```python
from build123d import *

# Parameters (mm, degrees)
BOSS_EXTRUDE1_DEPTH = 5
SKETCH2_R           = 11.25
CUT_EXTRUDE1_DEPTH  = 2.5
SKETCH3_R           = 1.5
SKETCH3_R_2         = 1
CUT_EXTRUDE3_DEPTH  = 12.5
CHAMFER1_SIZE       = 2.5
SKETCH5_R           = 5
CUT_EXTRUDE4_DEPTH  = 12.5


with BuildPart() as part:
    # Sketch1 → Boss-Extrude1 (new body)
    with BuildSketch(Plane(origin=(0, 0, 0), x_dir=(1, 0, 0), z_dir=(0, 1, 0))):
        Polygon((-65, 2.5), (-65, -17.5), (65, -17.5), (65, 2.5), (50, 17.5), (-50, 17.5), align=None)
    extrude(amount=BOSS_EXTRUDE1_DEPTH)

    # Sketch2 → Cut-Extrude1 (cut)
    with BuildSketch(Plane(origin=(0, 5, 0), x_dir=(1, 0, 0), z_dir=(0, 1, 0))):
        with Locations(Location((-42.5, 0, 0), (0, 0, 270))):
            Circle(SKETCH2_R)
        with Locations(Location((42.5, 0, 0), (0, 0, 90))):
            Circle(SKETCH2_R)
    extrude(amount=-CUT_EXTRUDE1_DEPTH, mode=Mode.SUBTRACT)

    # Sketch3 → Cut-Extrude3 (cut)
    with BuildSketch(Plane(origin=(0, 5, 0), x_dir=(1, 0, 0), z_dir=(0, 1, 0))):
        with Locations(Location((42.5, 0, 0), (0, 0, 270))):
            Circle(SKETCH3_R)
        with Locations(Location((42.5, 7.5, 0), (0, 0, 270))):
            Circle(SKETCH3_R_2)
        with Locations(Location((46, 7.5, 0), (0, 0, 270))):
            Circle(SKETCH3_R_2)
        with Locations(Location((39, 7.5, 0), (0, 0, 270))):
            Circle(SKETCH3_R_2)
        with Locations(Location((50, 3.5, 0), (0, 0, 270))):
            Circle(SKETCH3_R_2)
        with Locations(Location((50, 0, 0), (0, 0, 270))):
            Circle(SKETCH3_R_2)
        with Locations(Location((50, -3.5, 0), (0, 0, 270))):
            Circle(SKETCH3_R_2)
        with Locations(Location((46, -7.5, 0), (0, 0, 270))):
            Circle(SKETCH3_R_2)
        with Locations(Location((42.5, -7.5, 0), (0, 0, 270))):
            Circle(SKETCH3_R_2)
        with Locations(Location((39, -7.5, 0), (0, 0, 270))):
            Circle(SKETCH3_R_2)
        with Locations(Location((35, -3.5, 0), (0, 0, 270))):
            Circle(SKETCH3_R_2)
        with Locations(Location((35, 0, 0), (0, 0, 270))):
            Circle(SKETCH3_R_2)
        with Locations(Location((35, 3.5, 0), (0, 0, 270))):
            Circle(SKETCH3_R_2)
        with Locations(Location((-35, 3.5, 0), (0, 0, 270))):
            Circle(SKETCH3_R_2)
        with Locations(Location((-35, 0, 0), (0, 0, 270))):
            Circle(SKETCH3_R_2)
        with Locations(Location((-35, -3.5, 0), (0, 0, 270))):
            Circle(SKETCH3_R_2)
        with Locations(Location((-39, -7.5, 0), (0, 0, 270))):
            Circle(SKETCH3_R_2)
        with Locations(Location((-42.5, -7.5, 0), (0, 0, 270))):
            Circle(SKETCH3_R_2)
        with Locations(Location((-46, -7.5, 0), (0, 0, 270))):
            Circle(SKETCH3_R_2)
        with Locations(Location((-50, -3.5, 0), (0, 0, 270))):
            Circle(SKETCH3_R_2)
        with Locations(Location((-50, 0, 0), (0, 0, 270))):
            Circle(SKETCH3_R_2)
        with Locations(Location((-50, 3.5, 0), (0, 0, 270))):
            Circle(SKETCH3_R_2)
        with Locations(Location((-39, 7.5, 0), (0, 0, 270))):
            Circle(SKETCH3_R_2)
        with Locations(Location((-46, 7.5, 0), (0, 0, 270))):
            Circle(SKETCH3_R_2)
        with Locations(Location((-42.5, 7.5, 0), (0, 0, 270))):
            Circle(SKETCH3_R_2)
        with Locations(Location((-42.5, 0, 0), (0, 0, 270))):
            Circle(SKETCH3_R)
    extrude(amount=-CUT_EXTRUDE3_DEPTH, mode=Mode.SUBTRACT)

    # Chamfer1
    chamfer1_edges = [part.edges().sort_by_distance(p)[0] for p in [
        (57.5, 0, -10),
        (65, 0, 7.5),
        (65, 2.5, 17.5),
        (-65, 2.5, 17.5),
        (0, 0, 17.5),
        (-65, 0, 7.5),
        (-57.5, 0, -10),
        (0, 0, -17.5),
    ]]
    chamfer(chamfer1_edges, length=CHAMFER1_SIZE)

    # Sketch5 → Cut-Extrude4 (cut)
    with BuildSketch(Plane(origin=(0, 5, 0), x_dir=(1, 0, 0), z_dir=(0, 1, 0))):
        with Locations(Location((0, 0, 0), (0, 0, 270))):
            Circle(SKETCH5_R)
    extrude(amount=-CUT_EXTRUDE4_DEPTH, mode=Mode.SUBTRACT)


solid = part.part
```
Read the model definition and answer for the solid it produces. Units are mm, in the model's axes. A direction names the side the tool comes from. Round coordinates to 2 decimals unless told otherwise and drop trailing zeros. Write each loop counter-clockwise with the first axis right and the second up, starting at its lowest first coordinate (ties: lowest second). Pieces come first, ordered by that corner, then holes. Notation, with made-up numbers: (6, 43.25) -> (32, 43.25) arc R22 ccw to (32, 79.25) -> close; hole circle Ø2 at (36, 65). An arc over 180 degrees is marked (long way). Answer in a Markdown table with one row per item. Add a question column.
1) Which of the six approach directions +Z, -Z, +X, -X, +Y, -Y give full straight-line access (tool end or side, diameter ignored) to faces 5 (the face through (-1, 0, 6)), 6 (the face through (45, 2.5, 0))?
2) Find section C-C, the plane x = -16.5. Determine the outline of the cut face in (y, z), and give its area (3 significant figures).
3) Find section A-A, the plane x = 0. Determine the outline of the cut face in (y, z), and give its area (3 significant figures).
4) Given P1, Ø2.5, axis at x = -35, z = 3.5, coming from the +Y side; P2, Ø1, axis at y = 1, z = 7, coming from the +X side, each flat-ended and moving along its own axis, determine where each tip first touches the part or whether it passes through.
5) Determine the mould class of faces 1 (the face through (31.346, 3.768, 1.465)), 2 (the face through (-1, 1, 16)), 3 (the face through (-45, 2.5, 0)), 4 (the face through (-57.4, 3.7, -10.1)) for opening direction X: pulls with the +X half, pulls with the -X half, needs draft (parallel to the pull), parting line crosses it, or undercut.
6) Consider line 1 (X direction, y = 3.4, z = -0.5); line 2 (X direction, y = 4.2, z = -10); line 3 (X direction, y = 3.3, z = -7.5). Determine where each line is inside the solid, lowest interval first.
7) Find section B-B, the plane y = 4. Determine the outline of the cut face in (x, z), and give its area (4 significant figures).
Findings below:
| question | item | result |
|---|---|---|
| 1 | face 5 | +Z, -Z, +X, -X, -Y |
| 1 | face 6 | +Y |
| 2 | outline | (0, -15) -> (2.5, -17.5) -> (5, -17.5) -> (5, 17.5) -> (2.5, 17.5) -> (0, 15) -> close |
| 2 | area | 169 mm² |
| 3 | outline | (0, -15) -> (2.5, -17.5) -> (5, -17.5) -> (5, -5) -> (0, -5) -> close; (0, 5) -> (5, 5) -> (5, 17.5) -> (2.5, 17.5) -> (0, 15) -> close |
| 3 | area | 119 mm² |
| 4 | P1 | y = 2.5 |
| 4 | P2 | x = 64 |
| 5 | face 1 | undercut |
| 5 | face 2 | needs draft |
| 5 | face 3 | undercut |
| 5 | face 4 | pulls with the -X half |
| 6 | line 1 | -65 to -53.74, -31.26 to -4.97, 4.97 to 31.26, 53.74 to 65 |
| 6 | line 2 | -57.5 to -47.65, -37.35 to 37.35, 47.65 to 57.5 |
| 6 | line 3 | -60 to -50.89, -34.11 to 34.11, 50.89 to 60 |
| 7 | outline | (-65, -2.5) -> (-50, -17.5) -> (50, -17.5) -> (65, -2.5) -> (65, 15) -> (62.5, 17.5) -> (-62.5, 17.5) -> (-65, 15) -> close; hole circle Ø22.5 at (-42.5, 0); hole circle Ø10 at (0, 0); hole circle Ø22.5 at (42.5, 0) |
| 7 | area | 3,445 mm² |
